The listing builds one solid part. Answer for the finished solid, in the listing's coordinates (mm). A direction names the side the tool comes from. Give positions to 0.01 mm unless a question says otherwise; leave off trailing zeros. Loops run counter-clockwise (first coordinate to the right, second up) from the corner with the lowest first, then second, coordinate; pieces in that order, holes last. Notation, with made-up numbers: (73.25, 39) - (96.25, 39) arc R4 ccw to (96.25, 43) - close; hole circle Ø3 at (-7, -38). An arc over 180 degrees is marked (long way). Write each question's results on one line, items separated by ' | '.
Autodesk Inventor part; units mm, degrees
ref_plane "Work Plane1" through (-0.3969, -4.318, 2.3495) normal (1, 0, 0) x (0, 0, -1)
ref_plane "YZ Plane" through (0, 0, 0) normal (1, 0, 0) x (0, 1, 0)
ref_plane "XZ Plane" through (0, 0, 0) normal (0, 1, 0) x (-1, 0, 0)
sketch "Sketch1" plane through (0, 0, 0) normal (0, 0, 1) x (1, 0, 0)
  line L0 (-29.3688, -4.318) -> (-29.3688, 4.318)
  line L1 (-29.3688, 4.318) -> (29.3688, 4.318)
  line L2 (29.3688, 4.318) -> (29.3688, -4.318)
  line L3 (29.3688, -4.318) -> (1.5875, -4.318)
  line L4 (1.5875, -4.318) -> (1.5875, -1.143)
  line L5 (1.5875, -1.143) -> (-2.3812, -1.143)
  line L6 (-2.3812, -1.143) -> (-2.3812, -4.318)
  line L7 (-2.3812, -4.318) -> (-29.3688, -4.318)
  point P0 (0, 0)
  point P1 (0, 4.318)
  point P2 (-29.3688, 0)
  dimension "d0" = 58.7375
  dimension "d1" = 3.9688
  dimension "d2" = 3.175
  dimension "d3" = 27.7812
  dimension "d4" = 8.636
extrude "Extrusion1" add sketch "Sketch1" along normal mid plane 4.699
ref_plane "Work Plane1" through (-0.3969, -4.318, 2.3495) normal (1, 0, 0) x (0, 0, -1)
properties part number "Slide_Key" material "Steel, High Strength Low Alloy"
Item 1: A cutting plane is placed at B-B, the plane z = 1.05. Determine the outline of the cut face in (x, y).
Values found:
outline: (-29.37, -4.32) - (-2.38, -4.32) - (-2.38, -1.14) - (1.59, -1.14) - (1.59, -4.32) - (29.37, -4.32) - (29.37, 4.32) - (-29.37, 4.32) - close
Item 2: A cutting plane is placed at A-A, the plane y = -3.75. Determine the outline of the cut face in (x, z).
Values found:
outline: (-29.37, -2.35) - (-2.38, -2.35) - (-2.38, 2.35) - (-29.37, 2.35) - close; (1.59, -2.35) - (29.37, -2.35) - (29.37, 2.35) - (1.59, 2.35) - close
Item 3: A flat-ended cylindrical pin translates along its axis: P1, Ø1.2, axis at x = -1.5, z = 1, coming from the -Y side. Find the tip coordinate at first contact, or state that the pin passes through.
Values found:
P1: stops at y = -1.14
Item 4: For faces 1 (the face through (0, -1.143, 0)), 2 (the face through (0, 0, -2.35)), determine the directions among +Z, -Z, +X, -X, +Y, -Y from which every point of the face is accessible in a straight line to the end or side of a thin tool.
Values found:
face 1: +Z, -Z, -Y | face 2: -Z, +X, -X, +Y, -Y
Item 5: For a pull along X with two mould halves and no side action, classify faces 3 (the face through (29.369, 0, 0)), 4 (the face through (-2.381, -3, 0)), 5 (the face through (-16, -4.318, 0)) as released by +X, released by -X, zero draft, split by the parting line, or undercut.
Values found:
face 3: released by +X | face 4: undercut | face 5: zero draft
Item 6: Find the intervals of material crossed by line 1 along X through (y, z) = (-2.25, 1.1), in increasing order. Write a range as [from, to].
Values found:
line 1: x = [-29.37, -2.38], [1.59, 29.37]
